Autodesk Inventor part; units mm, degrees
ref_plane "YZ Plane" through (0, 0, 0) normal (1, 0, 0) x (0, 1, 0)
ref_plane "XZ Plane" through (0, 0, 0) normal (0, 1, 0) x (-1, 0, 0)
ref_plane "XY Plane" through (0, 0, 0) normal (0, 0, 1) x (1, 0, 0)
sketch "Sketch1" plane through (0, 0, 0) normal (0, 0, 1) x (1, 0, 0)
  line L0 (0, 0) -> (0, 203.2)
  line L1 (0, 203.2) -> (141.9905, 348.5579)
  line L2 (141.9905, 348.5579) -> (144.2617, 346.3393)
  line L3 (144.2617, 346.3393) -> (3.175, 201.9066)
  line L4 (3.175, 201.9066) -> (3.175, 0)
  line L5 (3.175, 0) -> (0, 0)
  dimension "d0" = 3.175
  dimension "d1" = 3.175
  dimension "d2" = 203.2
  dimension "d3" = 203.2
extrude "Extrusion1" add sketch "Sketch1" against normal blind 101.6
properties part number "backing"
CAD build for the part. Positions are in the model's coordinates, mm. A direction names the side the tool comes from. Give positions to 0.01 mm unless a question says otherwise; leave off trailing zeros. Loops run counter-clockwise (first coordinate to the right, second up) from the corner with the lowest first, then second, coordinate; pieces in that order, holes last. Notation, with made-up numbers: M 89.5,-34 L 136.5,-34 A28 ccw 136.5,-10 Z; hole C 40,25.5 d3. An arc over 180 degrees is marked long. One line per question, with ' | ' between items. Start each with the question number.
1. Probe L1, parallel to X at y = 182.5, z = -92 (3 decimals); L2, parallel to Y at x = 53.5, z = -71.5; L3, parallel to Y at x = 100, z = -68. List the from-to ranges inside material, lowest first. Write a range as from..to.
2. Saw through at C-C on x = 68. Give the cut face in (y, z).
3. 3-axis set-ups, long thin cutter, end or side, ignore diameter. For faces 1 (the face through (3.175, 102, -50)), 2 (the face through (2, 162, -101.6)): which of +Z, -Z, +X, -X, +Y, -Y reach the whole face in a straight line?
4. Saw through at A-A on z = -16. Give the cut face in (x, y) (1 decimal), plus the area to 3 significant figures.
5. Saw through at B-B on y = 302. Give the cut face in (x, z), plus the area to 3 significant figures.
6. Flat gauge pins, fed straight in: pin 1 (3 mm diameter, centred on y = 311, z = -61.5, fed in from -X); pin 2 (3 mm diameter, centred on x = 84.5, z = -39, fed in from -Y); pin 3 (1.5 mm diameter, centred on y = 58, z = -75, fed in from +X) (3 decimals). Where does each tip first touch, or does it go through?
Result sheet:
1) L1: x = 0..3.175 | L2: y = 253.43..257.97 | L3: y = 301.03..305.57
2) outline: M 268.27,-101.6 L 272.81,-101.6 L 272.81,0 L 268.27,0 Z
3) face 1: +Z, -Z, +X, -Y | face 2: -Z, +X, -X, +Y, -Y
4) outline: M 0,0 L 3.2,0 L 3.2,201.9 L 144.3,346.3 L 142,348.6 L 0,203.2 Z | area: 1,290 mm^2
5) outline: M 96.51,-101.6 L 100.95,-101.6 L 100.95,0 L 96.51,0 Z | area: 451 mm^2
6) pin 1: stops at x = 103.84 | pin 2: stops at y = 283.62 | pin 3: stops at x = 3.175
